CAD build for the part. Positions are in the model's coordinates, mm. A direction names the side the tool comes from. Give positions to 0.01 mm unless a question says otherwise; leave off trailing zeros. Write each loop counter-clockwise with the first axis right and the second up, starting at its lowest first coordinate (ties: lowest second). Pieces come first, ordered by that corner, then holes. Notation, with made-up numbers: (-33, 7.25) - (-18, 7.25) arc R18 ccw to (-18, 15.25) - close; hole circle Ø7 at (1, -6.75). An arc over 180 degrees is marked (long way). Answer as a JSON object with one key per item and string values.
from build123d import *

# Parameters (mm, degrees)
F0_R     = 1.4529433878
F0_W     = 5
F0_H     = 21.7857151878
F1_DEPTH = 5
F2_DEPTH = 30
F3_R     = 7.3585229381
F5_D     = 3
F5_DEPTH = 100
F5_TIP   = 0.9012909285
F6_D     = 3
F6_DEPTH = 100
F6_START = 15
F6_TIP   = 0.9012909285


with BuildPart() as f1:
    # F0 (on Top) → F1 (new body)
    with BuildSketch(Plane.XY):
        Polygon((46.8364858899, 15.218096768), (0, 49.2467956293), (-46.8364858899, 15.218096768), (-28.9465401936, -39.8414945826), (28.9465401936, -39.8414945826), align=None)
        with Locations((-26.0947393151, -35.9163274127)):
            Circle(F0_R, mode=Mode.SUBTRACT)
        with Locations((-17.5, 0)):
            Rectangle(F0_W, F0_H, mode=Mode.SUBTRACT)
        with Locations((26.0947393151, -35.9163274127)):
            Circle(F0_R, mode=Mode.SUBTRACT)
        with Locations((17.5, 0)):
            Rectangle(F0_W, F0_H, mode=Mode.SUBTRACT)
        with Locations((-42.2221751394, 13.7188163206)):
            Circle(F0_R, mode=Mode.SUBTRACT)
        with Locations((42.2221751394, 13.7188163206)):
            Circle(F0_R, mode=Mode.SUBTRACT)
        with Locations((0, 44.3950221842)):
            Circle(F0_R, mode=Mode.SUBTRACT)
    extrude(amount=F1_DEPTH)

    # F0 (on Top) → F2 (join)
    with BuildSketch(Plane.XY):
        with Locations((-17.5, 0)):
            Rectangle(F0_W, F0_H)
        with Locations((17.5, 0)):
            Rectangle(F0_W, F0_H)
    extrude(amount=F2_DEPTH)

    # F3
    f3_edges = [f1.edges().sort_by_distance(p)[0] for p in [
        (-17.5, -10.892858, 30),
        (17.5, -10.892858, 30),
        (17.5, 10.892858, 30),
        (-17.5, 10.892858, 30),
    ]]
    fillet(f3_edges, radius=F3_R)

    # F5 (one way)
    with BuildSketch(Plane(origin=(0, 0, 0), x_dir=(0, 1, 0), z_dir=(-1, 0, 0))):
        with Locations((0, -25)):
            Circle(F5_D / 2)
    extrude(amount=-F5_DEPTH, mode=Mode.SUBTRACT)
    with Locations(Plane(origin=(0, 0, 0), x_dir=(0, 1, 0), z_dir=(-1, 0, 0))):
        with Locations((0, -25)):
            with Locations((0, 0, -(F5_DEPTH + F5_TIP / 2))):  # 118° drill point
                Cone(0, F5_D / 2, F5_TIP, mode=Mode.SUBTRACT)

    # F6
    # its depths count from where the whole tool has entered the part; down to there all is cleared
    with Locations(Plane.YZ.offset(-F6_START)):
        with Locations((0, 25)):
            Hole(F6_D / 2, depth=F6_DEPTH)
            with Locations((0, 0, -(F6_DEPTH + F6_TIP / 2))):  # 118° drill point
                Cone(0, F6_D / 2, F6_TIP, mode=Mode.SUBTRACT)


solid = f1.part
(1) Probe L1, parallel to Z at x = 18.45, y = 0; L2, parallel to Z at x = -16.5, y = 31.5; L3, parallel to Z at x = 16, y = -1. List the from-to ranges inside material, lowest first. Write a range as [from, to].
Answer key:
{"L1": "z = [0, 23.5], [26.5, 30]", "L2": "z = [0, 5]", "L3": "z = [0, 23.88], [26.12, 30]"}
(2) Saw through at C-C, the plane z = 25. Give the cut face in (x, y), and give its area (3 significant figures).
Answer key:
{"outline": "(-20, -10.5) - (-15, -10.5) - (-15, -1.5) - (-20, -1.5) - close; (-20, 1.5) - (-15, 1.5) - (-15, 10.5) - (-20, 10.5) - close; (15, -10.5) - (20, -10.5) - (20, -1.5) - (15, -1.5) - close; (15, 1.5) - (20, 1.5) - (20, 10.5) - (15, 10.5) - close", "area": "180 mm²"}
(3) Saw through at B-B, the plane y = 0. Give the cut face in (x, z).
Answer key:
{"outline": "(-41.89, 0) - (41.89, 0) - (41.89, 5) - (20, 5) - (20, 23.5) - (15, 23.5) - (15, 5) - (-15, 5) - (-15, 23.5) - (-20, 23.5) - (-20, 5) - (-41.89, 5) - close; (-20, 26.5) - (-15, 26.5) - (-15, 30) - (-20, 30) - close; (15, 26.5) - (20, 26.5) - (20, 30) - (15, 30) - close"}
(4) Saw through at D-D, the plane x = 6.5. Give the cut face in (y, z).
Answer key:
{"outline": "(-39.84, 0) - (44.52, 0) - (44.52, 5) - (-39.84, 5) - close"}
(5) 3-axis set-ups, long thin cutter, end or side, ignore diameter. For faces 4 (the face through (-0.315, 42.977, 2.465)), 5 (the face through (20, 0, 17)), 6 (the face through (17.54, 8.79, 27.79)), 7 (the face through (-20, 0, 17)), 8 (the face through (17, -10.893, 14)): which of +Z, -Z, +X, -X, +Y, -Y reach the whole face in a straight line?
Answer key:
{"face 4": "+Z, -Z", "face 5": "+Z, +X, +Y, -Y", "face 6": "+Z, +X, -X, +Y", "face 7": "+Z, -X, +Y, -Y", "face 8": "+Z, +X, -X, -Y"}
(6) Saw through at A-A, the plane z = 13.25. Give the cut face in (x, y), and give its area (3 significant figures).
Answer key:
{"outline": "(-20, -10.89) - (-15, -10.89) - (-15, 10.89) - (-20, 10.89) - close; (15, -10.89) - (20, -10.89) - (20, 10.89) - (15, 10.89) - close", "area": "218 mm²"}
(7) Flat gauge pins, fed straight in: P1, Ø4, axis at x = 16.5, z = 12, coming from the -Y side; P2, Ø3.5, axis at x = -26.09, y = -35.92, coming from the +Z side; P3, Ø17.5, axis at y = 1, z = 18, coming from the -X side. Where does each tip first touch, or does it go through?
Answer key:
{"P1": "stops at y = -10.89", "P2": "stops at z = 5", "P3": "stops at x = -20"}
(8) Pull direction X, two halves, no side cores. Call faces 1 (the face through (-25.424, -37.205, 2.465)), 2 (the face through (-38.017, -11.926, 2.465)), 3 (the face through (-17.46, -8.68, 27.9)): pulls with the +X half, pulls with the -X half, needs draft (parallel to the pull), parting line crosses it, or undercut.
Answer key:
{"face 1": "undercut", "face 2": "pulls with the -X half", "face 3": "needs draft"}
